from build123d import *

# Parameters (mm, degrees)
BOSS_EXTRUDE1_DEPTH = 58.31
SKETCH3_R           = 2.5
CUT_EXTRUDE1_DEPTH  = 7.35
SKETCH4_R           = 2.5
CUT_EXTRUDE2_DEPTH  = 7.35
SKETCH5_W           = 25
SKETCH5_H           = 30
CUT_EXTRUDE3_DEPTH  = 59.31


with BuildPart() as part:
    # Sketch2 → Boss-Extrude1 (new body)
    with BuildSketch(Plane(origin=(0, 0, 0), x_dir=(1, 0, 0), z_dir=(0, 1, 0))):
        with BuildLine():
            Line((0, 0), (0, 30))
            Line((0, 30), (25, 30))
            Line((25, 30), (25, 23.65))
            Line((25, 23.65), (12.7, 23.65))
            ThreePointArc((12.7, 23.65), (8.209871939, 21.790128061), (6.35, 17.3))
            Line((6.35, 17.3), (6.35, 0))
            Line((6.35, 0), (0, 0))
        make_face()
    boss_extrude1 = extrude(amount=BOSS_EXTRUDE1_DEPTH)

    # Sketch3 → Cut-Extrude1 (cut, through all)
    with BuildSketch(Plane(origin=(6.35, 0, 0), x_dir=(0, 0, -1), z_dir=(1, 0, 0))):
        with Locations((8.65, 10)):
            Circle(SKETCH3_R)
        with Locations((8.65, 30)):
            Circle(SKETCH3_R)
    cut_extrude1 = extrude(amount=-CUT_EXTRUDE1_DEPTH, mode=Mode.SUBTRACT)

    # Sketch4 → Cut-Extrude2 (cut, through all)
    with BuildSketch(Plane.XY.offset(-23.65)):
        with Locations((18.706720962, 50.31)):
            Circle(SKETCH4_R)
    cut_extrude2 = extrude(amount=-CUT_EXTRUDE2_DEPTH, mode=Mode.SUBTRACT)

    # Mirror1: Boss-Extrude1, Cut-Extrude1, Cut-Extrude2 across plane
    add(boss_extrude1.mirror(Plane(origin=(0, 58.31, 0), x_dir=(1, 0, 0), z_dir=(0, 0, -1))))
    add(cut_extrude1.mirror(Plane(origin=(0, 58.31, 0), x_dir=(1, 0, 0), z_dir=(0, 0, -1))), mode=Mode.SUBTRACT)
    add(cut_extrude2.mirror(Plane(origin=(0, 58.31, 0), x_dir=(1, 0, 0), z_dir=(0, 0, -1))), mode=Mode.SUBTRACT)

    # Sketch5 → Cut-Extrude3 (cut, through all)
    with BuildSketch(Plane(origin=(0, 58.31, 0), x_dir=(1, 0, 0), z_dir=(0, 1, 0))):
        with Locations((12.5, 15)):
            Rectangle(SKETCH5_W, SKETCH5_H)
    extrude(amount=-CUT_EXTRUDE3_DEPTH, mode=Mode.SUBTRACT)


solid = part.part
Geometry: final body of the model. Coordinates: model frame, mm. A direction names the side the tool comes from. Coordinates: 2 decimals unless noted, no trailing zeros. Write each loop counter-clockwise with the first axis right and the second up, starting at its lowest first coordinate (ties: lowest second). Pieces come first, ordered by that corner, then holes. Notation, with made-up numbers: (-1.5, 72.25) - (45.5, 72.25) arc R32 cw to (45.5, 99.25) - close; hole circle Ø11 at (-29, 77). An arc over 180 degrees is marked (long way). Return JSON: item names as keys, results as strings.
Item 1: Section query A-A (y = 10). Output: boundary loops of the cut face in (x, z).
Completed:
{"outline": "(0, 0) - (6.35, 0) - (6.35, 6.15) - (0, 6.15) - close; (0, 11.15) - (6.35, 11.15) - (6.35, 17.3) arc R6.35 cw to (12.7, 23.65) - (25, 23.65) - (25, 30) - (0, 30) - close"}
Item 2: Reachability of faces 5 (the face through (19, 29, 23.65)), 6 (the face through (0, 29, 15)) from +Z, -Z, +X, -X, +Y, -Y: full face, straight path, thin tool, end or side. Return the list, or none.
Completed:
{"face 5": "-Z, +X, +Y, -Y", "face 6": "+Z, -Z, -X, +Y, -Y"}
Item 3: Line query: L1, parallel to Y at x = 3, z = 8.65; L2, parallel to X at y = 50.31, z = 27.75; L3, parallel to Z at x = 19.25, y = 5. Output: solid intervals per line, ascending.
Completed:
{"L1": "y = 0 to 7.5, 12.5 to 27.5, 32.5 to 58.31", "L2": "x = 0 to 16.21, 21.21 to 25", "L3": "z = 23.65 to 30"}
Item 4: Pull-direction query (Y, two-part tool) for faces 1 (the face through (18.16, 47.87, 26.78)), 2 (the face through (7, 0, 22)), 3 (the face through (7, 58.31, 22)), 4 (the face through (3, 30, 0)); classes: +Y half, -Y half, draft (parallel to the pull), parting line (faces both ways), or undercut.
Completed:
{"face 1": "undercut", "face 2": "-Y half", "face 3": "+Y half", "face 4": "draft"}
Item 5: Section query D-D (x = 18.5). Output: boundary loops of the cut face in (y, z), and give its area (3 significant figures).
Completed:
{"outline": "(0, 23.65) - (47.82, 23.65) - (47.82, 30) - (0, 30) - close; (52.8, 23.65) - (58.31, 23.65) - (58.31, 30) - (52.8, 30) - close", "area": "339 mm2"}
Item 6: Pin query (flat end, axial travel): pin 1 Ø8 at (y, z) = (10, 8.65) entering from +X; pin 2 Ø8 at (y, z) = (30, 8.65) entering from +X; pin 3 Ø13.5 at (x, y) = (19, 33) entering from -Z. Return the tip coordinate at first contact, or that it passes through.
Completed:
{"pin 1": "stops at x = 6.35", "pin 2": "stops at x = 6.35", "pin 3": "stops at z = 23.63"}
Item 7: Section query B-B (z = 8.65). Output: boundary loops of the cut face in (x, y).
Completed:
{"outline": "(0, 0) - (6.35, 0) - (6.35, 7.5) - (0, 7.5) - close; (0, 12.5) - (6.35, 12.5) - (6.35, 27.5) - (0, 27.5) - close; (0, 32.5) - (6.35, 32.5) - (6.35, 58.31) - (0, 58.31) - close"}
Item 8: Section query C-C (x = 2.25). Output: boundary loops of the cut face in (y, z).
Completed:
{"outline": "(0, 0) - (58.31, 0) - (58.31, 30) - (0, 30) - close; hole circle Ø5 at (10, 8.65); hole circle Ø5 at (30, 8.65)"}
